Autodesk Inventor part; units mm, degrees
ref_plane "YZ Plane" through (0, 0, 0) normal (1, 0, 0) x (0, 1, 0)
ref_plane "XZ Plane" through (0, 0, 0) normal (0, 1, 0) x (-1, 0, 0)
ref_plane "XY Plane" through (0, 0, 0) normal (0, 0, 1) x (1, 0, 0)
sketch "Sketch1" plane through (0, 0, 0) normal (0, 1, 0) x (-1, 0, 0)
  line L0 (606, 0) -> (606, -30)
  arc A0 (557.4011, -115.7783) -> (606, -30) centre (506, -30) ccw
  arc A1 (0, -270) -> (557.4011, -115.7783) centre (0, 814.4143) ccw
  line L1 (0, 191.6842) -> (0, -191.6842)
  arc A2 (0, -264) -> (554.3171, -110.6316) centre (0, 814.4143) ccw
  arc A3 (554.3171, -110.6316) -> (600, -30) centre (506, -30) ccw
  line L2 (600, -30) -> (600, 0)
  line L3 (600, 0) -> (606, 0)
  line L4 (0, -264) -> (0, -270)
  point P0 (0, 0)
  point P1 (0, 0)
  point P2 (0, -267)
  point P3 (0, -163.7009)
  point P4 (0, -169.7009)
  dimension "d0" = 100
  dimension "d1" = 30
  dimension "d3" = 1084.4143
  dimension "d6" = 6
  dimension "d11" = 1200
  dimension "d12" = 270
revolve "Revolution1" add sketch "Sketch1" angle 360 about axis through (0, 0, 191.6842) along (0, 0, -1)
sketch "Sketch2" plane through (0, 0, 0) normal (0, 0, 1) x (1, 0, 0)
  circle A0 centre (0, 0) radius 16.75
  dimension "d8" = 33.5
extrude "Extrusion1" cut sketch "Sketch2" against normal through all
equation "\"Disherd_head_hight\" = d12"
properties part number "PNV - 704 dished head D1200" material "Steel"
The model under review builds one solid part; all positions refer to its coordinate system, in mm. Round coordinates to 2 decimals unless told otherwise and drop trailing zeros.
Item 1: For line 1 (Y direction, x = 0, z = -16.5); line 2 (X direction, y = 21, z = -156); line 3 (Y direction, x = -203, z = -156.5), list the stretches that pass through material, from the lowest coordinate up.
Determined:
line 1: y = -606 to -600, 600 to 606
line 2: x = -483.54 to -469.93, 469.93 to 483.54
line 3: y = -438.26 to -423.19, 423.19 to 438.26
Item 2: Clearance check with flat-ended pins moving along their axes: pin 1 Ø3 at (x, y) = (-14, 368.5) entering from -Z; pin 2 Ø1.5 at (y, z) = (44, -106.5) entering from +X; pin 3 Ø2 at (y, z) = (-222.5, -60.5) entering from +X. State where each tip first meets the part, or that it passes through.
Determined:
pin 1: stops at z = -205.91
pin 2: stops at x = 569.59
pin 3: stops at x = 559.07
Item 3: Mouldability with a two-part tool opening along Y and no side actions: class faces 1 (the face through (78.108, -594.894, -14.79)), 2 (the face through (586, 137, 0)), 3 (the face through (605.414, 26.645, -15.21)), 4 (the face through (-3.63, -16.35, -266.83)) as released by +Y, released by -Y, zero draft, split by the parting line, or undercut.
Determined:
face 1: undercut
face 2: zero draft
face 3: split by the parting line
face 4: undercut
